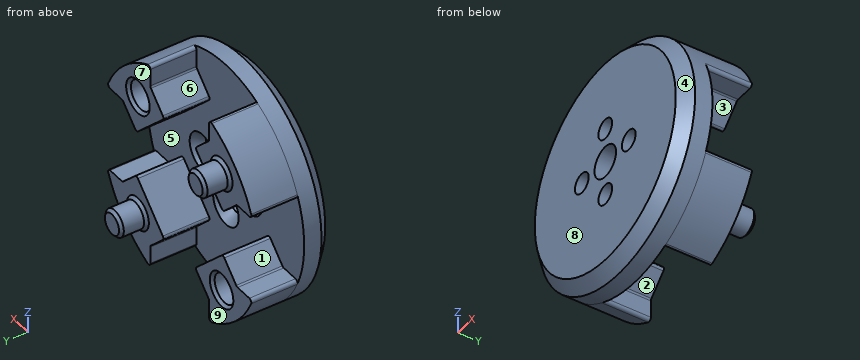
```python
from build123d import *
from OCP.BRepFilletAPI import BRepFilletAPI_MakeChamfer

# Parameters (mm, degrees)
SKETCH_1_R                             = 20
EXTRUDE_1_DEPTH                        = 5
EXTRUDE_2_DEPTH                        = 8
FILLET_1_R                             = 0.5
PATTERN_START                          = 5
PATTERN_CIRCULAR_1_DEPTH               = 8
SKETCH_3_R                             = 2.5000000000000004
CUT_EXTRUDE_1_DEPTH                    = 5
EXTRUDE_START                          = 4.5
SKETCH_3_3_R                           = 2.5000000000000004
SKETCH_3_3_R_2                         = 2.2999999999999994
EXTRUDE_3_DEPTH                        = 4.5
CHAMFER_1_SIZE                         = 0.5
SKETCH_4_R                             = 2.75
CUT_EXTRUDE_2_DEPTH                    = 34.26033673912518
CHAMFER_2_SIZE                         = 2
CUT_EXTRUDE_3_REACH                    = 32.923
SKETCH_5_R                             = 1.75
CHAMFER_3_SIZE2                        = 1.787630389
CHAMFER_3_SIZE                         = 1.5
PATTERN_CIRCULAR_2_COUNT               = 4
CHAMFER_3_OF_PATTERN_CIRCULAR_2_SIZE   = 1.5
CHAMFER_3_OF_PATTERN_CIRCULAR_2_SIZE_2 = 1.787630389
CHAMFER_4_SIZE                         = 1


# Read off the part's stored shape, not the designer's step: 阵列(圆周)1
# Some blends are built 0.0001 mm under size
with BuildPart() as part:
    # 草图1 → 凸台-拉伸1 (new body)
    with BuildSketch(Plane(origin=(0, 0, 0), x_dir=(1, 0, 0), z_dir=(0, 1, 0))):
        with Locations(Location((0, 0, 0), (0, 0, 270))):
            Circle(SKETCH_1_R)
    extrude(amount=EXTRUDE_1_DEPTH)

    # 草图2 → 凸台-拉伸2 (add)
    with BuildSketch(Plane(origin=(0, 5, 0), x_dir=(1, 0, 0), z_dir=(0, 1, 0))):
        with BuildLine():
            Line((14.57106781186547, -7.500000000000001), (11.035533905932741, -3.9644660940672627))
            Line((11.035533905932741, -3.9644660940672627), (3.9644660940672627, -11.03553390593274))
            Line((3.9644660940672627, -11.03553390593274), (7.500000000000001, -14.571067811865477))
            Line((7.500000000000001, -14.571067811865477), (7.500000000000001, -18.540496217739157))
            ThreePointArc((7.500000000000001, -18.540496217739157), (14.142135623730951, -14.14213562373095), (18.540496217739157, -7.500000000000001))
            Line((18.540496217739157, -7.500000000000001), (14.57106781186547, -7.500000000000001))
        make_face()
    extrude(amount=EXTRUDE_2_DEPTH)

    # 圆角1
    fillet_1_edges = [part.edges().sort_by_distance(p)[0] for p in [
        (7.500000000000001, 9, 14.571067811865477),
        (7.500000000000001, 9, 18.540496217739157),
        (18.540496217739154, 9, 7.500000000000002),
        (14.57106781186547, 9, 7.500000000000001),
        (11.035533905932741, 9, 3.9644660940672627),
        (3.9644660940672627, 9, 11.03553390593274),
    ]]
    fillet(fillet_1_edges, radius=FILLET_1_R)

    # 阵列(圆周)1 outline → 阵列(圆周)1 (add)
    with BuildSketch(Plane(origin=(0, 0, 0), x_dir=(1, 0, 0), z_dir=(0, 1, 0)).offset(PATTERN_START)):
        with BuildLine():
            ThreePointArc((17.783419244, 7.5), (18.203278805, 7.728489505), (18.239404353, 8.205128205))
            ThreePointArc((18.239404353, 8.205128205), (14.142135624, 14.142135624), (8.205128205, 18.239404353))
            ThreePointArc((8.205128205, 18.239404353), (7.728489505, 18.203278805), (7.5, 17.783419244))
            Line((7.5, 17.783419244), (7.5, 14.778174593))
            ThreePointArc((7.5, 14.778174593), (7.461939766, 14.586832877), (7.353553391, 14.424621202))
            Line((7.353553391, 14.424621202), (4.318019485, 11.389087297))
            ThreePointArc((4.318019485, 11.389087297), (4.171572875, 11.035533906), (4.318019485, 10.681980515))
            Line((4.318019485, 10.681980515), (10.681980515, 4.318019485))
            ThreePointArc((10.681980515, 4.318019485), (11.035533906, 4.171572875), (11.389087297, 4.318019485))
            Line((11.389087297, 4.318019485), (14.424621202, 7.353553391))
            ThreePointArc((14.424621202, 7.353553391), (14.586832877, 7.461939766), (14.778174593, 7.5))
            Line((14.778174593, 7.5), (17.783419244, 7.5))
        make_face()
        with BuildLine():
            ThreePointArc((-18.239404353, -8.205128205), (-14.142135624, -14.142135624), (-8.205128205, -18.239404353))
            ThreePointArc((-8.205128205, -18.239404353), (-7.728489505, -18.203278805), (-7.5, -17.783419244))
            Line((-7.5, -17.783419244), (-7.5, -14.778174593))
            ThreePointArc((-7.5, -14.778174593), (-7.461939766, -14.586832877), (-7.353553391, -14.424621202))
            Line((-7.353553391, -14.424621202), (-4.318019485, -11.389087297))
            ThreePointArc((-4.318019485, -11.389087297), (-4.171572875, -11.035533906), (-4.318019485, -10.681980515))
            Line((-4.318019485, -10.681980515), (-10.681980515, -4.318019485))
            ThreePointArc((-10.681980515, -4.318019485), (-11.035533906, -4.171572875), (-11.389087297, -4.318019485))
            Line((-11.389087297, -4.318019485), (-14.424621202, -7.353553391))
            ThreePointArc((-14.424621202, -7.353553391), (-14.586832877, -7.461939766), (-14.778174593, -7.5))
            Line((-14.778174593, -7.5), (-17.783419244, -7.5))
            ThreePointArc((-17.783419244, -7.5), (-18.203278805, -7.728489505), (-18.239404353, -8.205128205))
        make_face()
        with BuildLine():
            ThreePointArc((-7.5, 17.783419244), (-7.728489505, 18.203278805), (-8.205128205, 18.239404353))
            ThreePointArc((-8.205128205, 18.239404353), (-14.142135624, 14.142135624), (-18.239404353, 8.205128205))
            ThreePointArc((-18.239404353, 8.205128205), (-18.203278805, 7.728489505), (-17.783419244, 7.5))
            Line((-17.783419244, 7.5), (-14.778174593, 7.5))
            ThreePointArc((-14.778174593, 7.5), (-14.586832877, 7.461939766), (-14.424621202, 7.353553391))
            Line((-14.424621202, 7.353553391), (-11.389087297, 4.318019485))
            ThreePointArc((-11.389087297, 4.318019485), (-11.035533906, 4.171572875), (-10.681980515, 4.318019485))
            Line((-10.681980515, 4.318019485), (-4.318019485, 10.681980515))
            ThreePointArc((-4.318019485, 10.681980515), (-4.171572875, 11.035533906), (-4.318019485, 11.389087297))
            Line((-4.318019485, 11.389087297), (-7.353553391, 14.424621202))
            ThreePointArc((-7.353553391, 14.424621202), (-7.461939766, 14.586832877), (-7.5, 14.778174593))
            Line((-7.5, 14.778174593), (-7.5, 17.783419244))
        make_face()
    extrude(amount=PATTERN_CIRCULAR_1_DEPTH)

    # 草图3 → 切除-拉伸1 (cut)
    with BuildSketch(Plane(origin=(0, 13.000000000000002, 0), x_dir=(1, 0, 0), z_dir=(0, 1, 0))):
        with Locations(Location((-10.681980515339466, 10.681980515339463, 0), (0, 0, 270))):
            Circle(SKETCH_3_R)
        with Locations(Location((10.681980515339466, -10.681980515339463, 0), (0, 0, 270))):
            Circle(SKETCH_3_R)
    extrude(amount=-CUT_EXTRUDE_1_DEPTH, mode=Mode.SUBTRACT)

    # 草图3<3> → 凸台-拉伸3 (add)
    with BuildSketch(Plane(origin=(0, 13.000000000000002, 0), x_dir=(1, 0, 0), z_dir=(0, 1, 0)).offset(EXTRUDE_START)):
        with Locations(Location((10.681980515339466, -10.681980515339463, 0), (0, 0, 270))):
            Circle(SKETCH_3_3_R)
        with Locations(Location((-10.681980515339466, 10.681980515339463, 0), (0, 0, 270))):
            Circle(SKETCH_3_3_R)
        with Locations(Location((10.681980515339466, 10.681980515339463, 0), (0, 0, 270))):
            Circle(SKETCH_3_3_R_2)
        with Locations(Location((-10.681980515339465, -10.681980515339465, 0), (0, 0, 270))):
            Circle(SKETCH_3_3_R_2)
    extrude(amount=-EXTRUDE_3_DEPTH)


with BuildPart() as extrude_3_kept_piece:
    # of the separate pieces the step leaves, the one the design keeps (extrude_3_pieces_kept)
    add(part.part.solids().sort_by_distance((8.205128205, 5, 18.239404353))[0])

    # 倒角1
    chamfer_1_edges = [extrude_3_kept_piece.edges().sort_by_distance(p)[0] for p in [
        (-10.681980515339466, 8.000000000000002, -13.181980515339463),
        (-10.681980515339466, 13.000000000000002, -13.181980515339463),
        (10.681980515339466, 8.000000000000002, 8.181980515339463),
        (10.681980515339466, 13.000000000000002, 8.181980515339463),
        (10.681980515339466, 13.000000000000002, -12.981980515339462),
        (10.681980515339466, 17.5, -12.981980515339462),
        (-10.681980515339465, 13.000000000000002, 8.381980515339466),
        (-10.681980515339465, 17.5, 8.381980515339466),
    ]]
    chamfer(chamfer_1_edges, length=CHAMFER_1_SIZE)

    # 草图4 → 切除-拉伸2 (cut, through all)
    with BuildSketch(Plane.XZ):
        with Locations(Location((0, 0, 0), (0, 0, 270))):
            Circle(SKETCH_4_R)
    extrude(amount=-CUT_EXTRUDE_2_DEPTH, mode=Mode.SUBTRACT)

    # 倒角2
    chamfer_2_edges = [extrude_3_kept_piece.edges().sort_by_distance(p)[0] for p in [
        (6.12e-15, 0, -20),
    ]]
    chamfer(chamfer_2_edges, length=CHAMFER_2_SIZE)

    # 草图5 → 切除-拉伸3 (cut, up to next)
    with BuildSketch(Plane(origin=(0, 5, 0), x_dir=(1, 0, 0), z_dir=(0, 1, 0)), mode=Mode.PRIVATE) as cut_extrude_3_sk1:
        with Locations(Location((6, 0, 0), (0, 0, 270))):
            Circle(SKETCH_5_R)
    cut_extrude_3_tool1 = extrude(cut_extrude_3_sk1.sketch, amount=-CUT_EXTRUDE_3_REACH, mode=Mode.PRIVATE) & extrude_3_kept_piece.part
    cut_extrude_3 = cut_extrude_3_tool1.solids().sort_by_distance((6, 5, 0))[0]
    add(cut_extrude_3, mode=Mode.SUBTRACT)

    # 倒角3
    chamfer_3_edges = [extrude_3_kept_piece.edges().sort_by_distance(p)[0] for p in [
        (6.000000000000001, 5, -1.75),
    ]]
    chamfer_3_side = [extrude_3_kept_piece.faces().sort_by_distance(p)[0] for p in [
        (6.000000000000001, 5, -1.78),
    ]]
    chamfer(chamfer_3_edges, length=CHAMFER_3_SIZE - 0.0001, length2=CHAMFER_3_SIZE2 - 0.0001, reference=chamfer_3_side[0])  # a hair under: the kernel refuses the full size

    # 阵列(圆周)2: 切除-拉伸3 ×4 about axis
    pattern_circular_2_axis = Axis((0, 0, -1.047e-14), (0, 1, 0))
    for i in range(1, PATTERN_CIRCULAR_2_COUNT):
        add(cut_extrude_3.rotate(pattern_circular_2_axis, i * 360 / PATTERN_CIRCULAR_2_COUNT), mode=Mode.SUBTRACT)

    # 倒角3 of 阵列(圆周)2
    chamfer_3_of_pattern_circular_2_edges_1 = [extrude_3_kept_piece.edges().sort_by_distance(p)[0] for p in [
        (-1.749999999999989, 5, -6.0000000000000115),
    ]]
    chamfer_3_of_pattern_circular_2_side_1 = [extrude_3_kept_piece.faces().sort_by_distance(p)[0] for p in [
        (-1.779999999999989, 5, -6.0000000000000115),
    ]]
    chamfer_3_of_pattern_circular_2_edges_2 = [extrude_3_kept_piece.edges().sort_by_distance(p)[0] for p in [
        (-6.000000000000001, 5, 1.7499999999999785),
    ]]
    chamfer_3_of_pattern_circular_2_side_2 = [extrude_3_kept_piece.faces().sort_by_distance(p)[0] for p in [
        (-6.000000000000001, 5, 1.7799999999999785),
    ]]
    chamfer_3_of_pattern_circular_2_edges_3 = [extrude_3_kept_piece.edges().sort_by_distance(p)[0] for p in [
        (1.7499999999999882, 5, 5.99999999999999),
    ]]
    chamfer_3_of_pattern_circular_2_side_3 = [extrude_3_kept_piece.faces().sort_by_distance(p)[0] for p in [
        (1.7799999999999883, 5, 5.99999999999999),
    ]]
    chamfer_3_of_pattern_circular_2 = BRepFilletAPI_MakeChamfer(extrude_3_kept_piece.part.solid().wrapped)
    for e in chamfer_3_of_pattern_circular_2_edges_1:
        chamfer_3_of_pattern_circular_2.Add(CHAMFER_3_OF_PATTERN_CIRCULAR_2_SIZE - 0.0001, CHAMFER_3_OF_PATTERN_CIRCULAR_2_SIZE_2 - 0.0001, e.wrapped, chamfer_3_of_pattern_circular_2_side_1[0].wrapped)
    for e in chamfer_3_of_pattern_circular_2_edges_2:
        chamfer_3_of_pattern_circular_2.Add(CHAMFER_3_OF_PATTERN_CIRCULAR_2_SIZE - 0.0001, CHAMFER_3_OF_PATTERN_CIRCULAR_2_SIZE_2 - 0.0001, e.wrapped, chamfer_3_of_pattern_circular_2_side_2[0].wrapped)
    for e in chamfer_3_of_pattern_circular_2_edges_3:
        chamfer_3_of_pattern_circular_2.Add(CHAMFER_3_OF_PATTERN_CIRCULAR_2_SIZE - 0.0001, CHAMFER_3_OF_PATTERN_CIRCULAR_2_SIZE_2 - 0.0001, e.wrapped, chamfer_3_of_pattern_circular_2_side_3[0].wrapped)
    add(Compound.cast(chamfer_3_of_pattern_circular_2.Shape()), mode=Mode.REPLACE)  # a hair under: the kernel refuses the full size

    # 倒角4
    # the kernel refuses this chamfer: 1 mm, written as the material it takes off along each edge
    with BuildSketch(Plane(origin=(0, 5, 0), x_dir=(-1.8e-16, 0, -1), z_dir=(-1, 0, 1.8e-16))) as chamfer_4_piece_1:
        Polygon((2.75 + CHAMFER_4_SIZE, 0), (2.75, CHAMFER_4_SIZE), (2.75, 0), align=None)
    revolve(axis=Axis((0, 5, 0), (0, -1, 0)), mode=Mode.SUBTRACT)


solid = extrude_3_kept_piece.part
```
Geometry: final body of the model. Coordinates: model frame, mm. Face numbers are marked on the shaded views. A direction names the side the tool comes from. Round coordinates to 2 decimals unless told otherwise and drop trailing zeros. Order: outer loops, then holes, each group sorted by start corner. A loop starts at its lowest first (then second) coordinate and runs counter-clockwise, first axis right, second up. Notation, with made-up numbers: (51, 59.5) -> (98, 59.5) arc R4 ccw to (98, 65.5) -> close; hole circle Ø4 at (-25, 1.5). An arc over 180 degrees is marked (long way). Use one line per item in the form item = value. Start each with the question number.
1. Draft query along Z for the marked faces 1, 2, 3 and 4. Return one class per face: pulls with the +Z half, pulls with the -Z half, needs draft (parallel to the pull), parting line crosses it, or undercut.
2. Line query: probe 1 along X at (y, z) = (1.35, 0); probe 2 along Z at (x, y) = (12, 8.75); probe 3 along Y at (x, z) = (2.5, -13.5). Output: solid intervals per line, ascending.
3. Pin query (flat end, axial travel): pin 1 Ø2 at (y, z) = (9.5, 11) entering from -X; pin 2 Ø8 at (x, z) = (-8.5, 12.5) entering from -Y; pin 3 Ø2.5 at (y, z) = (7, 17) entering from +X; pin 4 Ø1.5 at (x, y) = (17, 9.5) entering from +Z. Return the tip coordinate at first contact, or that it passes through.
4. Cut plane A-A (z = 0). Return the cut outline in (x, y).
5. Cut plane B-B (y = 1.5). Return the cut outline in (x, z), then the cut area to 3 significant figures.
6. Reachability of the marked faces 5, 6, 7, 8 and 9 from +Z, -Z, +X, -X, +Y, -Y: full face, straight path, thin tool, end or side. Return the list, or none.
7. Cut plane C-C (x = 0). Return the cut outline in (y, z), then the cut area to 3 significant figures.
Solution:
q1.face_1 = undercut
q1.face_2 = pulls with the -Z half
q1.face_3 = undercut
q1.face_4 = parting line crosses it
q2.probe_1 = -19.35 to -7.75, -4.25 to -2.75, 2.75 to 4.25, 7.75 to 19.35
q2.probe_2 = -16 to -4.93, 4.93 to 8.56, 12.81 to 16
q2.probe_3 = 0 to 5
q3.pin_1 = -17.32
q3.pin_2 = 0
q3.pin_3 = 12.33
q3.pin_4 = 11.66
q4.outline = (-20, 2) -> (-18, 0) -> (-7.75, 0) -> (-7.75, 3.21) -> (-9.25, 5) -> (-20, 5) -> close; (-4.25, 0) -> (-2.75, 0) -> (-2.75, 4) -> (-3.21, 4.46) -> (-4.25, 3.21) -> close; (2.75, 0) -> (4.25, 0) -> (4.25, 3.21) -> (3.21, 4.46) -> (2.75, 4) -> close; (7.75, 0) -> (18, 0) -> (20, 2) -> (20, 5) -> (9.25, 5) -> (7.75, 3.21) -> close
q5.outline = circle Ø39 at (0, 0); hole circle Ø3.5 at (-6, 0); hole circle Ø5.5 at (0, 0); hole circle Ø3.5 at (0, -6); hole circle Ø3.5 at (0, 6); hole circle Ø3.5 at (6, 0)
q5.area = 1,130 mm^2
q6.face_5 = +Y
q6.face_6 = +Z, +Y
q6.face_7 = +Z, +X, +Y
q6.face_8 = +Z, -Z, +X, -X, -Y
q6.face_9 = -Z, -X, +Y
q7.outline = (0, -18) -> (2, -20) -> (5, -20) -> (5, -9.25) -> (3.21, -7.75) -> (0, -7.75) -> close; (0, -4.25) -> (3.21, -4.25) -> (4.46, -3.21) -> (4, -2.75) -> (0, -2.75) -> close; (0, 2.75) -> (4, 2.75) -> (4.46, 3.21) -> (3.21, 4.25) -> (0, 4.25) -> close; (0, 7.75) -> (3.21, 7.75) -> (5, 9.25) -> (5, 20) -> (2, 20) -> (0, 18) -> close
q7.area = 128 mm^2
